Geometry: final body of the model. Coordinates: model frame, mm. Face numbers are marked on the shaded views. A direction names the side the tool comes from. Give positions to 0.01 mm unless a question says otherwise; leave off trailing zeros. Order: outer loops, then holes, each group sorted by start corner. A loop starts at its lowest first (then second) coordinate and runs counter-clockwise, first axis right, second up. Notation, with made-up numbers: (-33.75, 57.25) - (16.25, 57.25) arc R5 ccw to (16.25, 64.25) - close; hole circle Ø1 at (69, 26.25). An arc over 180 degrees is marked (long way). Put each result on its own line as item: value. Start each with the question number.
1. Section A-A on z = 20.32. Count the separate pieces of the cut face and the enclosed holes in it, plus the area to 3 significant figures.
2. Section B-B on x = 17.5. Return the cut outline in (y, z) (3 decimals).
3. Ray query, line 1 along X through (y, z) = (-4.2, 20.32); line 2 along X through (y, z) = (8, 24); line 3 along Y through (x, z) = (19, 20.5). Return the intervals inside material, ascending. Write a range as from..to.
4. Set-up query: the marked faces 4, 5 and 6. Return all of +Z, -Z, +X, -X, +Y, -Y with unobstructed straight access to the full face (end or side cutting, diameter ignored); none if empty.
5. Section C-C on x = 8.25. Return the cut outline in (y, z) (3 decimals), plus the area to 3 significant figures.
6. First-contact query: P1, Ø4.5, axis at x = 24.5, z = 21, coming from the +Y side (3 decimals); P2, Ø5, axis at y = -2, z = 19.5, coming from the -X side; P3, Ø4.5, axis at y = 17.5, z = 19, coming from the -X side. Flat tips, straight axial feed; report the tip coordinate or a pass-through.
7. Mould query, pull axis X, two halves, no side actions, for the marked faces 1, 2 and 3. Classes: pulls with the +X half, pulls with the -X half, needs draft (parallel to the pull), parting line crosses it, or undercut.
from build123d import *

# Parameters (mm, degrees)
SKETCH1_R                = 2.38125
BOSS_EXTRUDE1_DEPTH      = 38.1
FILLET1_R                = 6.35
SKETCH3_W                = 38.1
SKETCH3_H                = 6.35
BOSS_EXTRUDE2_DEPTH      = 12.7
SKETCH2_W                = 7.62
SKETCH2_H                = 8.89
CUT_EXTRUDE7_DEPTH       = 66.019560197
BOSS_EXTRUDE5_DEPTH      = 22.225
BOSS_EXTRUDE5_DEPTH_BACK = 9.525
SKETCH10_W               = 7.62
SKETCH10_H               = 8.89
CUT_EXTRUDE1_DEPTH       = 62.376176621
CUT_EXTRUDE1_DEPTH_BACK  = 62.376176621
SKETCH5_R                = 1.905
SKETCH6_W                = 8.89
SKETCH6_H                = 8.89
BOSS_EXTRUDE4_DEPTH      = 3.175
CUT_EXTRUDE2_DEPTH       = 71.485759779
CUT_EXTRUDE2_DEPTH_BACK  = 71.485759779
SKETCH7_R                = 2.0828
CUT_EXTRUDE8_DEPTH       = 13.335
CUT_EXTRUDE9_DEPTH       = 62.376176621
SKETCH12_W               = 15.875
SKETCH12_H               = 6.35
CUT_EXTRUDE10_DEPTH      = 40.128574278


with BuildPart() as part:
    # Sketch1 → Boss-Extrude1 (new body)
    with BuildSketch(Plane.XY):
        with BuildLine():
            Line((-37.385625, -8.255), (-37.385625, -3.175))
            Line((-37.385625, -3.175), (-37.385625, 3.175))
            Line((-37.385625, 3.175), (37.385625, 3.175))
            Line((37.385625, 3.175), (37.385625, -3.175))
            Line((37.385625, -3.175), (-27.543125, -3.175))
            Line((-27.543125, -3.175), (-27.543125, -8.255))
            ThreePointArc((-27.543125, -8.255), (-32.464375, -13.17625), (-37.385625, -8.255))
        make_face()
        with Locations(Location((-32.464375, -8.255, 0), (0, 0, 180))):
            Circle(SKETCH1_R, mode=Mode.SUBTRACT)
    extrude(amount=BOSS_EXTRUDE1_DEPTH)

    # Fillet1
    fillet1_edges = [part.edges().sort_by_distance(p)[0] for p in [
        (-37.385625, 3.175, 19.05),
    ]]
    fillet(fillet1_edges, radius=FILLET1_R)

    # Sketch3 → Boss-Extrude2 (add)
    with BuildSketch(Plane(origin=(37.385625, 0, 0), x_dir=(0, 0, -1), z_dir=(1, 0, 0))):
        with Locations((-19.05, 0)):
            Rectangle(SKETCH3_W, SKETCH3_H)
    extrude(amount=BOSS_EXTRUDE2_DEPTH)

    # Sketch2 → Cut-Extrude7 (cut, through all)
    with BuildSketch(Plane(origin=(0, 3.175, 0), x_dir=(1, 0, 0), z_dir=(0, 1, 0))):
        with Locations((17.541875, -20.32)):
            Rectangle(SKETCH2_W, SKETCH2_H)
    extrude(amount=-CUT_EXTRUDE7_DEPTH, mode=Mode.SUBTRACT)

    # Sketch10 → Boss-Extrude5 (add, two sides: drawn at the far end of the back side and taken through both)
    with BuildSketch(Plane(origin=(0, 3.175, 0), x_dir=(1, 0, 0), z_dir=(0, 1, 0)).offset(-BOSS_EXTRUDE5_DEPTH_BACK)):
        with Locations((17.541875, -20.32)):
            Rectangle(SKETCH10_W, SKETCH10_H)
    extrude(amount=BOSS_EXTRUDE5_DEPTH + BOSS_EXTRUDE5_DEPTH_BACK)

    # Sketch5 → Cut-Extrude1 (cut, two sides: drawn at the far end of the back side and taken through both)
    with BuildSketch(Plane.XY.offset(24.765).offset(-CUT_EXTRUDE1_DEPTH_BACK)):
        with Locations((17.541875, 5.715)):
            Circle(SKETCH5_R)
        with Locations((17.541875, 23.1775)):
            Circle(SKETCH5_R)
    extrude(amount=CUT_EXTRUDE1_DEPTH + CUT_EXTRUDE1_DEPTH_BACK, mode=Mode.SUBTRACT)

    # Sketch6 → Boss-Extrude4 (add)
    with BuildSketch(Plane(origin=(0, -3.175, 0), x_dir=(1, 0, 0), z_dir=(0, 1, 0))):
        with Locations((9.286875, -20.32)):
            Rectangle(SKETCH6_W, SKETCH6_H)
        with Locations((25.796875, -20.32)):
            Rectangle(SKETCH6_W, SKETCH6_H)
    extrude(amount=-BOSS_EXTRUDE4_DEPTH)

    # Sketch7 → Cut-Extrude2 (cut, two sides: drawn at the far end of the back side and taken through both)
    with BuildSketch(Plane(origin=(0, -6.35, 0), x_dir=(-1, 0, 0), z_dir=(0, -1, 0)).offset(-CUT_EXTRUDE2_DEPTH_BACK)):
        with Locations(Location((-9.286875, -20.32, 0), (0, 0, 90))):
            Circle(SKETCH7_R)
        with Locations(Location((-25.796875, -20.32, 0), (0, 0, 90))):
            Circle(SKETCH7_R)
    extrude(amount=CUT_EXTRUDE2_DEPTH + CUT_EXTRUDE2_DEPTH_BACK, mode=Mode.SUBTRACT)

    # Sketch9 → Cut-Extrude8 (cut)
    with BuildSketch(Plane.XY.offset(38.1)):
        with BuildLine():
            Line((50.085625, 3.175), (50.085625, -3.175))
            Line((50.085625, -3.175), (-27.543125, -3.175))
            Line((-27.543125, -3.175), (-27.543125, -8.255))
            ThreePointArc((-27.543125, -8.255), (-32.464375, -13.17625), (-37.385625, -8.255))
            Line((-37.385625, -8.255), (-37.385625, -3.175))
            ThreePointArc((-37.385625, -3.175), (-35.525753061, 1.315128061), (-31.035625, 3.175))
            Line((-31.035625, 3.175), (50.085625, 3.175))
        make_face()
    extrude(amount=-CUT_EXTRUDE8_DEPTH, mode=Mode.SUBTRACT)

    # Sketch11 → Cut-Extrude9 (cut, through all)
    with BuildSketch(Plane.XY.offset(24.765)):
        Polygon((21.351875, 3.175), (21.351875, -3.175), (30.241875, -3.175), (54.982981917, -12.803682108), (51.254802373, 20.663231938), align=None)
        Polygon((4.841875, -3.175), (13.731875, -3.175), (13.731875, 3.175), (-41.256071428, 5.663811912), (-38.308208532, -22.514289292), align=None)
    extrude(amount=-CUT_EXTRUDE9_DEPTH, mode=Mode.SUBTRACT)

    # Sketch12 → Cut-Extrude10 (cut, through all)
    with BuildSketch(Plane(origin=(21.351875, 0, 0), x_dir=(0, 0, -1), z_dir=(1, 0, 0))):
        with Locations((-7.9375, 0)):
            Rectangle(SKETCH12_W, SKETCH12_H)
    extrude(amount=-CUT_EXTRUDE10_DEPTH, mode=Mode.SUBTRACT)


solid = part.part
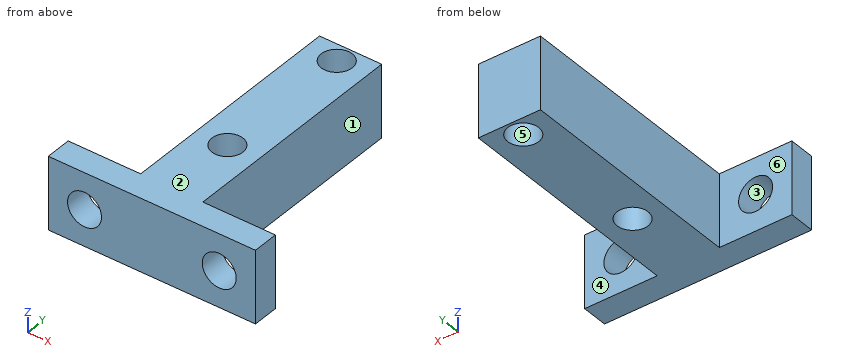
Resolved:
1. separate pieces: 3
1. enclosed holes: 2
1. area: 249 mm^2
2. outline: (-6.35, 15.875) - (3.81, 15.875) - (3.81, 24.765) - (-6.35, 24.765) - close; (7.62, 15.875) - (21.273, 15.875) - (21.273, 24.765) - (7.62, 24.765) - close; (25.082, 15.875) - (25.4, 15.875) - (25.4, 24.765) - (25.082, 24.765) - close
3. line 1: 4.84..7.2, 11.37..23.71, 27.88..30.24
3. line 2: 13.73..21.35
3. line 3: -6.35..4.49, 6.94..21.95, 24.4..25.4
4. face 4: +Z, -Z, +X, +Y
4. face 5: +Z, -Z
4. face 6: +Z, -Z, -X, +Y
5. outline: (-6.35, 15.875) - (-3.175, 15.875) - (-3.175, 18.514) - (-6.35, 18.514) - close; (-6.35, 22.126) - (-3.175, 22.126) - (-3.175, 24.765) - (-6.35, 24.765) - close
5. area: 16.8 mm^2
6. P1: y = -3.175
6. P2: x = 4.84
6. P3: x = 13.73
7. face 1: pulls with the +X half
7. face 2: needs draft
7. face 3: undercut
